from build123d import *

# Parameters (mm, degrees)
F3_DEPTH       = 2.4765
F4_R           = 1.27
F5_DEPTH       = 17.272
F6_R           = 1.27
F7_DEPTH       = 13.462
F8_R           = 1.0434793425
F9_DEPTH       = 95.7072
F9_DEPTH_BACK  = 132
F10_R          = 0.3833262894
F11_DEPTH      = 32.2036075046
F11_DEPTH_BACK = 66.8030001


# Not quite as in the source:
# - an extrude ends at something that could not be found from the text; its depth is read off the source's solid


with BuildPart() as f1:
    # F0 (on Front) → F1 (revolve)
    with BuildSketch(Plane.XZ):
        with BuildLine():
            Line((63.5, 1.0541), (0, 1.0541))
            Line((0, 1.0541), (0, 0))
            Line((0, 0), (66.802, 0))
            add(Edge.make_bspline(
                [(63.5, 1.0541), (64.35611099, 1.0419137543), (66.7864059348, 0.5992812803), (66.802, 0)],
                knots=[0, 0, 0, 0, 3.4661694722, 3.4661694722, 3.4661694722, 3.4661694722], degree=3))
        make_face()
    revolve(axis=Axis((33.401, 0, 0), (1, 0, 0)))

    # F2 (on Front) → F3 (join, symmetric)
    with BuildSketch(Plane.XZ):
        Polygon((0.0045924954, 3.0420540417), (-14.9306075046, 3.0420540417), (-14.9306075046, -2.7999459583), (-13.4860288486, -6.8151904523), (2.3921924954, -3.8408457662), align=None)
    extrude(amount=F3_DEPTH, both=True)

    # F4 (on face) → F5 (join)
    with BuildSketch(Plane(origin=(-14.9306075046, 0, 0), x_dir=(0, -1, 0), z_dir=(-1, 0, 0))):
        Circle(F4_R)
    extrude(amount=F5_DEPTH)

    # F6 (on face) → F7 (join)
    with BuildSketch(Plane(origin=(-14.1114148908, 0, -5.0769134453), x_dir=(0, -1, 0), z_dir=(-0.9409553089, 0, -0.3385308062))):
        with Locations((0, 0.2862465809)):
            Circle(F6_R)
    extrude(amount=F7_DEPTH)

    # F8 (on face) → F9 (cut, two sides)
    with BuildSketch(Plane(origin=(-32.2026075046, 0, 0), x_dir=(0, -1, 0), z_dir=(-1, 0, 0))) as f9_sk:
        Circle(F8_R)
    extrude(amount=-F9_DEPTH, mode=Mode.SUBTRACT)
    extrude(f9_sk.sketch, amount=F9_DEPTH_BACK, mode=Mode.SUBTRACT)

    # F10 (on Right) → F11 (cut, two sides)
    with BuildSketch(Plane.YZ) as f11_sk:
        Circle(F10_R)
    extrude(amount=-F11_DEPTH, mode=Mode.SUBTRACT)
    extrude(f11_sk.sketch, amount=F11_DEPTH_BACK, mode=Mode.SUBTRACT)


solid = f1.part
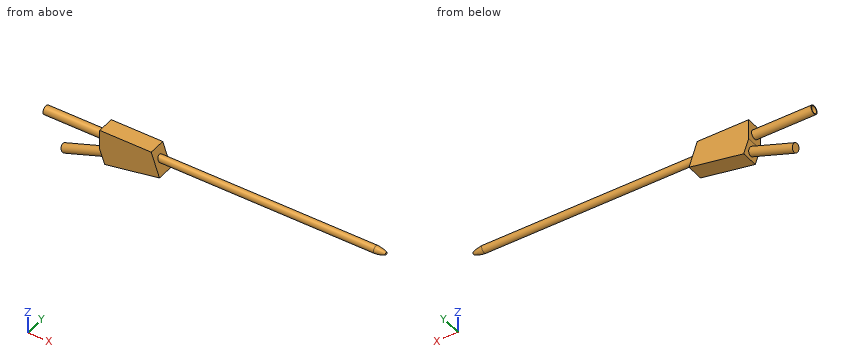
The listing builds one solid part. Answer for the finished solid, in the listing's coordinates (mm). Give positions to 0.01 mm unless a question says otherwise; leave off trailing zeros. Loops run counter-clockwise (first coordinate to the right, second up) from the corner with the lowest first, then second, coordinate; pieces in that order, holes last.
Item 1: Find the intervals of material crossed by line 1 along X through (y, z) = (-0.3, 2); line 2 along Y through (x, z) = (64.2, 0); line 3 along Y through (x, z) = (-24.5, -0.75), in increasing order.
Derived:
line 1: x = -14.93 to 0.37
line 2: y = -0.99 to -0.38, 0.38 to 0.99
line 3: y = -1.02 to -0.73, 0.73 to 1.02
Item 2: Each of these flat-tipped pins is pushed along its axis until it touches: pin 1 Ø1 at (y, z) = (0.5, 0) entering from -X; pin 2 Ø2 at (y, z) = (2, -2.5) entering from +X; pin 3 Ø2 at (x, y) = (8, 1.5) entering from -Z. Where does it stop, or does it pass through?
Derived:
pin 1: stops at x = 63.5
pin 2: stops at x = 2.27
pin 3: stops at z = -0.93
Item 3: A cutting plane is placed at A-A (x = -6). Give the vertices of the cut face in (y, z), then the cut area to 3 significant figures.
Derived:
outline: (-2.48, -5.41) - (2.48, -5.41) - (2.48, 3.04) - (-2.48, 3.04) - close; hole circle Ø2.09 at (0, 0)
area: 38.5 mm2
